Geometry check sheet. Reference: the model listing, model coordinates, mm. Face numbers are marked on the shaded views. Coordinates: 2 decimals unless noted, no trailing zeros. Write each loop counter-clockwise with the first axis right and the second up, starting at its lowest first coordinate (ties: lowest second). Pieces come first, ordered by that corner, then holes. Notation, with made-up numbers: M 69,39.25 L 89,39.25 A28 cw 89,67.25 Z; hole C -40,-32.5 d2. An arc over 180 degrees is marked long. Put each result on its own line as item: value. Start each with the question number.
1) Gauge pin test, flat ends, axial feed: pin 1 (3 mm diameter, centred on x = 21.5, y = 9, fed in from -Z); pin 2 (1.1 mm diameter, centred on x = 18.5, y = 0.5, fed in from -Z); pin 3 (0.8 mm diameter, centred on y = 0.5, z = -2, fed in from +X). Record the tip position at first contact, or that the pin passes through.
2) Cross-section at A-A on z = 0. Count the separate pieces of the cut face and the enclosed holes in it, plus the area to 3 significant figures.
3) Cross-section at C-C on y = 10.75. Record the cut outline in (x, z).
4) Mould release check, pull along Z, two halves, no side actions. Record for the marked faces 1, 2 and 3: released by +Z, released by -Z, zero draft, split by the parting line, or undercut.
5) Scan lines: line 1 along X through (y, z) = (10.5, 0); line 2 along Y through (x, z) = (5.5, -26); line 3 along Z through (x, y) = (-3, 12.75). Record each from-to range of solid material in increasing order.
from build123d import *

# Parameters (mm, degrees)
CROQUIS1_R              = 35
SALIENTE_EXTRUIR1_DEPTH = 15
CROQUIS2_R              = 34
CORTAR_EXTRUIR1_DEPTH   = 14
REDONDEO1_R             = 0.5
REDONDEO5_R             = 0.5
CORTAR_EXTRUIR2_REACH   = 53.72
CROQUIS3_W              = 5.5
CROQUIS3_H              = 14.4
CROQUIS3_W_2            = 7.5
CROQUIS3_H_2            = 16


with BuildPart() as part:
    # Croquis1 → Saliente-Extruir1 (new body)
    with BuildSketch(Plane(origin=(0, 0, 0), x_dir=(1, 0, 0), z_dir=(0, 1, 0))):
        with Locations(Location((0, 0, 0), (0, 0, 270))):
            Circle(CROQUIS1_R)
    extrude(amount=SALIENTE_EXTRUIR1_DEPTH)

    # Croquis2 → Cortar-Extruir1 (cut)
    with BuildSketch(Plane(origin=(0, 15, 0), x_dir=(1, 0, 0), z_dir=(0, 1, 0))):
        with Locations(Location((0, 0, 0), (0, 0, 270))):
            Circle(CROQUIS2_R)
    extrude(amount=-CORTAR_EXTRUIR1_DEPTH, mode=Mode.SUBTRACT)

    # Redondeo1
    redondeo1_edges = [part.edges().sort_by_distance(p)[0] for p in [
        (0, 0, -35),
    ]]
    fillet(redondeo1_edges, radius=REDONDEO1_R)

    # Redondeo5
    redondeo5_edges = [part.edges().sort_by_distance(p)[0] for p in [
        (0, 15, -35),
        (0, 15, -34),
        (0, 1, -34),
    ]]
    fillet(redondeo5_edges, radius=REDONDEO5_R - 0.0001)  # a hair under: the kernel refuses the full size

    # Croquis3 → Cortar-Extruir2 (cut, up to next)
    with BuildSketch(Plane.XZ, mode=Mode.PRIVATE) as cortar_extruir2_sk1:
        with Locations((20, 0)):
            Rectangle(CROQUIS3_W, CROQUIS3_H)
    cortar_extruir2_tool1 = extrude(cortar_extruir2_sk1.sketch, amount=-CORTAR_EXTRUIR2_REACH, mode=Mode.PRIVATE) & part.part
    # Croquis3 → Cortar-Extruir2 (cut, up to next)
    with BuildSketch(Plane.XZ, mode=Mode.PRIVATE) as cortar_extruir2_sk2:
        with Locations((-20, 0)):
            Rectangle(CROQUIS3_W_2, CROQUIS3_H_2)
    cortar_extruir2_tool2 = extrude(cortar_extruir2_sk2.sketch, amount=-CORTAR_EXTRUIR2_REACH, mode=Mode.PRIVATE) & part.part
    add(cortar_extruir2_tool1.solids().sort_by_distance((20, 0, 0))[0], mode=Mode.SUBTRACT)
    add(cortar_extruir2_tool2.solids().sort_by_distance((-20, 0, 0))[0], mode=Mode.SUBTRACT)


solid = part.part
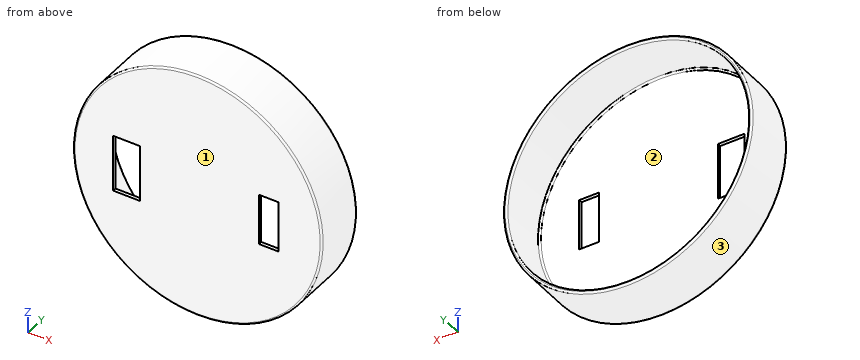
Answer key:
1. pin 1: stops at z = -28.72
1. pin 2: stops at z = -30.05
1. pin 3: stops at x = 34.96
2. separate pieces: 3
2. enclosed holes: 0
2. area: 84.8 mm²
3. outline: C 0,0 d70; hole C 0,0 d68
4. face 1: zero draft
4. face 2: undercut
4. face 3: split by the parting line
5. line 1: x = -35 to -34, 34 to 35
5. line 2: y = 0 to 1
5. line 3: z = -34.87 to -33.87, 33.87 to 34.87
